CAD build for the part. Positions are in the model's coordinates, mm. A direction names the side the tool comes from. Coordinates: 2 decimals unless noted, no trailing zeros. Order: outer loops, then holes, each group sorted by start corner. A loop starts at its lowest first (then second) coordinate and runs counter-clockwise, first axis right, second up. Notation, with made-up numbers: M 80.5,77 L 136.5,77 A9 cw 136.5,87 Z; hole C 65.25,-24.75 d9. An arc over 180 degrees is marked long. One line per item, written item: value.
from build123d import *

# Parameters (mm, degrees)
SKETCH_1_W          = 100
SKETCH_1_H          = 70
SKETCH_1_R          = 1
SKETCH_1_R_2        = 6.5
EXTRUDE_2_DEPTH     = 1.2
SKETCH_2_W          = 47
SKETCH_2_H          = 12.1
CUT_EXTRUDE_1_DEPTH = 106.954896064
SKETCH_4_R          = 15
CUT_EXTRUDE_2_DEPTH = 0.2
CUT_EXTRUDE_4_DEPTH = 106.954896064
FILLET_3_R          = 15
CUT_EXTRUDE_6_DEPTH = 106.954896064


with BuildPart() as part:
    # ｽｹｯﾁ1 → ﾎﾞｽ - 押し出し2 (new body)
    with BuildSketch(Plane(origin=(0, 0, 0), x_dir=(0, 1, 0), z_dir=(0, 0, 1))):
        with Locations((-50, 0)):
            Rectangle(SKETCH_1_W, SKETCH_1_H)
        with Locations(Location((-25.147606065, 20.2, 0), (0, 0, 270))):
            Circle(SKETCH_1_R, mode=Mode.SUBTRACT)
        with Locations(Location((-50.167606065, 20.2, 0), (0, 0, 270))):
            Circle(SKETCH_1_R, mode=Mode.SUBTRACT)
        with Locations(Location((-25.147606065, -20.2, 0), (0, 0, 270))):
            Circle(SKETCH_1_R, mode=Mode.SUBTRACT)
        with Locations(Location((-50.167606065, -20.2, 0), (0, 0, 270))):
            Circle(SKETCH_1_R, mode=Mode.SUBTRACT)
        with Locations(Location((-63.441664971, 0, 0), (0, 0, 270))):
            Circle(SKETCH_1_R_2, mode=Mode.SUBTRACT)
        with Locations(Location((-81.5344254, 0, 0), (0, 0, 270))):
            Circle(SKETCH_1_R, mode=Mode.SUBTRACT)
    extrude(amount=-EXTRUDE_2_DEPTH)

    # ｽｹｯﾁ2 → ｶｯﾄ - 押し出し1 (cut, through all)
    with BuildSketch(Plane(origin=(0, 0, 0), x_dir=(0, 1, 0), z_dir=(0, 0, 1))):
        with Locations((-37.657606065, 28.95)):
            Rectangle(SKETCH_2_W, SKETCH_2_H)
        with Locations((-37.657606065, -28.95)):
            Rectangle(SKETCH_2_W, SKETCH_2_H)
    extrude(amount=-CUT_EXTRUDE_1_DEPTH, mode=Mode.SUBTRACT)

    # ｽｹｯﾁ4 → ｶｯﾄ - 押し出し2 (cut)
    with BuildSketch(Plane.XY):
        with Locations((0, -63.441664971)):
            Circle(SKETCH_4_R)
    extrude(amount=-CUT_EXTRUDE_2_DEPTH, mode=Mode.SUBTRACT)

    # ｽｹｯﾁ7 → ｶｯﾄ - 押し出し4 (cut, through all)
    with BuildSketch(Plane.XY):
        Polygon((-35, -85.857864376), (-20.857864376, -100), (-35, -100), align=None)
        Polygon((35, -85.857864376), (35, -100), (20.857864376, -100), align=None)
    extrude(amount=-CUT_EXTRUDE_4_DEPTH, mode=Mode.SUBTRACT)

    # ﾌｨﾚｯﾄ3
    fillet_3_edges = [part.edges().sort_by_distance(p)[0] for p in [
        (-35, -85.857864376, -0.6),
        (-20.857864376, -100, -0.6),
        (20.857864376, -100, -0.6),
        (35, -85.857864376, -0.6),
    ]]
    fillet(fillet_3_edges, radius=FILLET_3_R)

    # ｽｹｯﾁ11 → ｶｯﾄ - 押し出し6 (cut, through all)
    with BuildSketch(Plane.XY):
        Polygon((31.822624011, -77.576242792), (28.844985556, -77.941850822), (28.479377526, -74.964212367), (31.45701598, -74.598604337), align=None)
        Polygon((15.82016764, -91.78479944), (13.222091429, -93.28479944), (14.722091429, -95.882875652), (17.32016764, -94.382875652), align=None)
        Polygon((-31.45701598, -74.598604337), (-28.479377526, -74.964212367), (-28.844985556, -77.941850822), (-31.822624011, -77.576242792), align=None)
        Polygon((-14.722091429, -95.882875652), (-17.32016764, -94.382875652), (-15.82016764, -91.78479944), (-13.222091429, -93.28479944), align=None)
    extrude(amount=-CUT_EXTRUDE_6_DEPTH, mode=Mode.SUBTRACT)


solid = part.part
Q1. Slice it at B-B (x = 9). List the corners of the cut face in (y, z).
Recorded:
outline: M -100,-1.2 L 0,-1.2 L 0,0 L -51.44,0 L -51.44,-0.2 L -75.44,-0.2 L -75.44,0 L -100,0 Z
Q2. Drill centre lines: line 1 along Y through (x, z) = (-20.2, -0.7); line 2 along X through (y, z) = (-94, -0.3); line 3 along X through (y, z) = (-24, -0.55). Where is each one in solid material? Low to high.
Recorded:
line 1: y = -98.93 to -51.17, -49.17 to -26.15, -24.15 to 0
line 2: x = -26.86 to -17.1, -13.64 to 13.64, 17.1 to 26.86
line 3: x = -22.9 to 22.9
Q3. Slice it at D-D (z = -0.8). Give the number of separate pieces and of enclosed holes in the cut face, plus the area to 3 significant figures.
Recorded:
separate pieces: 1
enclosed holes: 10
area: 5,460 mm^2
Q4. Pin check, flat tips, straight feed: pin 1 Ø1.2 at (x, y) = (20.2, -50.17) entering from -Z; pin 2 Ø6 at (x, y) = (-0.5, -58) entering from +Z; pin 3 Ø15 at (x, y) = (0, -63.44) entering from -Z; pin 4 Ø0.6 at (y, z) = (-46, -0.5) entering from -X. Stop position of each tip, or through.
Recorded:
pin 1: passes through
pin 2: stops at z = -0.2
pin 3: stops at z = -1.2
pin 4: stops at x = -22.9
Q5. Which spindle directions (+Z, -Z, +X, -X, +Y, -Y) get a long thin tool onto all of the face, cutting with end or side? Do faces 1 (the face through (-19.739, -26.035, -0.592)), 2 (the face through (6, -67, -0.2)). Say none if no direction does.
Recorded:
face 1: +Z, -Z
face 2: +Z
Q6. Slice it at A-A (x = 0). List the corners of the cut face in (y, z), plus the area to 3 significant figures.
Recorded:
outline: M -100,-1.2 L -82.53,-1.2 L -82.53,0 L -100,0 Z; M -80.53,-1.2 L -69.94,-1.2 L -69.94,-0.2 L -78.44,-0.2 L -78.44,0 L -80.53,0 Z; M -56.94,-1.2 L 0,-1.2 L 0,0 L -48.44,0 L -48.44,-0.2 L -56.94,-0.2 Z
area: 98.6 mm^2
Q7. Slice it at C-C (y = -55). List the corners of the cut face in (x, z).
Recorded:
outline: M -22.9,-1.2 L 22.9,-1.2 L 22.9,0 L 12.4,0 L 12.4,-0.2 L -12.4,-0.2 L -12.4,0 L -22.9,0 Z
Q8. Mould opens along Y. For faces 3 (the face through (-20.31, -98.89, -0.61)), 4 (the face through (-8.3, -50.7, 0)), 5 (the face through (-0.846, -56.997, -0.693)) say: released by +Y, released by -Y, zero draft, split by the parting line, or undercut.
Recorded:
face 3: released by -Y
face 4: zero draft
face 5: undercut
